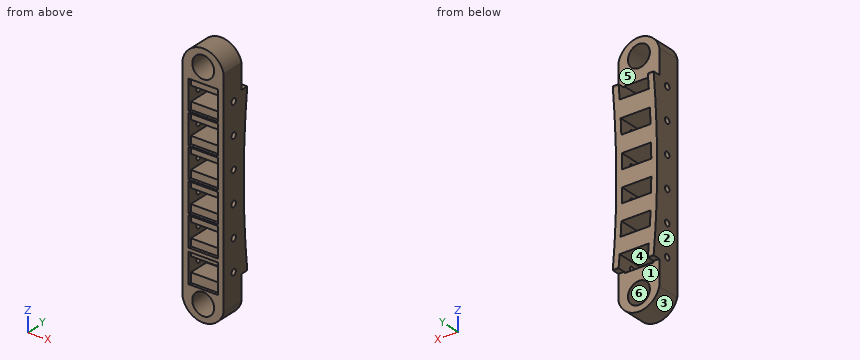
Autodesk Inventor part; units mm, degrees
ref_plane "Work Plane1" through (0, 8.9795, -42.5) normal (0, 1, 0) x (-1, 0, 0)
ref_plane "YZ Plane" through (0, 0, 0) normal (1, 0, 0) x (0, 1, 0)
ref_plane "XY Plane" through (0, 0, 0) normal (0, 0, 1) x (1, 0, 0)
sketch "Sketch1" plane through (0, 0, 0) normal (1, 0, 0) x (0, 1, 0)
  line L0 (0, 0) -> (0, -85)
  line L1 (0, -85) -> (8, -85)
  line L2 (0, 0) -> (8, 0)
  line L3 (8, 0) -> (8, -14)
  line L4 (8, -85) -> (8, -71)
  line L5 (8, -14) -> (9, -14)
  line L6 (8, -71) -> (9, -71)
  arc A0 (10.5, -14.5) -> (10.5, -70.5) centre (267.5593, -42.5) ccw
  line L7 (8, -71) -> (10.555, -71)
  line L8 (8, -14) -> (10.555, -14)
  arc A1 (10.555, -14) -> (10.555, -71) centre (267.5473, -42.5) ccw
extrude "Extrusion1" add sketch "Sketch1" along normal mid plane 14
sketch "Sketch2" plane through (-7, 8, 0) normal (0, 1, 0) x (1, 0, 0)
  line L0 (0, 85) -> (0, 0)
  line L1 (0, 14.0338) -> (0, 5.5338)
  line L2 (14, 0) -> (14, 85)
  line L3 (14, 14.0338) -> (14, 5.5338)
  arc A0 (0, 5.5338) -> (14, 5.5338) centre (7, 7.1942) ccw
  line L4 (0, 5.5338) -> (0, 0)
  line L5 (0, 0) -> (14, 0)
  line L6 (14, 0) -> (14, 5.5338)
  point P0 (7, 0)
  dimension "d13" = 8.5
extrude "Extrusion2" cut sketch "Sketch2" against normal blind 14
sketch "Sketch3" plane through (-7, 8, -71) normal (0, 1, 0) x (1, 0, 0)
  line L0 (0, 0) -> (14, 0)
  line L1 (0, 0) -> (0, 14)
  arc A0 (14, 8.5) -> (0, 8.5) centre (7, 6.7955) ccw
  line L2 (0, 8.5) -> (0, 14)
  line L3 (0, 14) -> (14, 14)
  line L4 (14, 14) -> (14, 8.5)
  line L5 (14, -65.4662) -> (14, 14)
  line L6 (0, 14) -> (0, 8.5)
  line L7 (14, 8.5) -> (14, 14)
  line L8 (14, 14) -> (0, 14)
  line L9 (0, 8.5) -> (0, 14)
  line L10 (0, 14) -> (14, 14)
  line L11 (14, 14) -> (14, 8.5)
  line L12 (14, 14) -> (14, 0)
  arc A1 (14, 8.5) -> (0, 8.5) centre (7, 6.7955) ccw
  point P0 (7, -71)
extrude "Extrusion3" cut sketch "Sketch3" against normal blind 14 contours L1 L3 A0 | A0 L3 L4
sketch "Sketch7" plane through (0, 0, -7.1942) normal (0, -1, 0) x (1, 0, 0)
  circle A0 centre (0, 2.1942) radius 3
  line L0 (0, -0.8058) -> (0, -3.8058)
  circle A1 centre (0, -72.0142) radius 1.5
  line L1 (0, -70.5142) -> (0, -67.5142)
  line L2 (0, -67.5142) -> (-5, -67.5142)
  line L3 (-5, -67.5142) -> (5, -67.5142)
  line L4 (-5, -67.5142) -> (5, -67.5142)
  line L5 (5, -67.5142) -> (5, -57.4342)
  line L6 (5, -57.4342) -> (-5, -57.4342)
  line L7 (-5, -57.4342) -> (-5, -67.5142)
  line L8 (0, -57.4342) -> (0, -56.9342)
  line L9 (-5, -56.2258) -> (5, -56.2258)
  line L10 (5, -56.2258) -> (5, -46.1458)
  line L11 (5, -46.1458) -> (-5, -46.1458)
  line L12 (-5, -46.1458) -> (-5, -56.2258)
  line L13 (0, -46.1458) -> (0, -45.6458)
  line L14 (-5, -45.6458) -> (5, -45.6458)
  line L15 (5, -45.6458) -> (5, -35.5658)
  line L16 (5, -35.5658) -> (-5, -35.5658)
  line L17 (-5, -35.5658) -> (-5, -45.6458)
  line L18 (0, -35.5658) -> (0, -35.0658)
  line L19 (-5, -35.0658) -> (5, -35.0658)
  line L20 (5, -35.0658) -> (5, -24.9858)
  line L21 (5, -24.9858) -> (-5, -24.9858)
  line L22 (-5, -24.9858) -> (-5, -35.0658)
  line L23 (0, -24.9858) -> (0, -24.4858)
  line L24 (-5, -24.4858) -> (5, -24.4858)
  line L25 (5, -24.4858) -> (5, -14.4058)
  line L26 (5, -14.4058) -> (-5, -14.4058)
  line L27 (-5, -14.4058) -> (-5, -24.4858)
  line L28 (0, -14.4058) -> (0, -13.9058)
  line L29 (-5, -13.9058) -> (5, -13.9058)
  line L30 (5, -13.9058) -> (5, -3.8058)
  line L31 (5, -3.8058) -> (-5, -3.8058)
  line L32 (-5, -3.8058) -> (-5, -13.9058)
  point P0 (0, 7.1942)
extrude "Extrusion6" cut sketch "Sketch7" against normal blind 1 contours L31 L30 L29 L32 | L2 L7 L6 L5 L3
sketch "Sketch8" plane through (0, 0, -7.1942) normal (0, -1, 0) x (1, 0, 0)
  line L0 (-5, -57.4342) -> (5, -57.4342)
  line L1 (0, -57.4342) -> (0, -56.9342)
  line L2 (-5, -56.2258) -> (5, -56.2258)
  line L3 (5, -56.2258) -> (5, -46.1458)
  line L4 (5, -46.1458) -> (-5, -46.1458)
  line L5 (-5, -46.1458) -> (-5, -56.2258)
  line L6 (0, -46.1458) -> (0, -45.6458)
  line L7 (-5, -45.6458) -> (5, -45.6458)
  line L8 (5, -45.6458) -> (5, -35.5658)
  line L9 (5, -35.5658) -> (-5, -35.5658)
  line L10 (-5, -35.5658) -> (-5, -45.6458)
  line L11 (0, -35.5658) -> (0, -35.0658)
  line L12 (-5, -35.0658) -> (5, -35.0658)
  line L13 (5, -35.0658) -> (5, -24.9858)
  line L14 (5, -24.9858) -> (-5, -24.9858)
  line L15 (-5, -24.9858) -> (-5, -35.0658)
  line L16 (0, -24.9858) -> (0, -24.4858)
  line L17 (-5, -24.4858) -> (5, -24.4858)
  line L18 (5, -24.4858) -> (5, -14.4058)
  line L19 (5, -14.4058) -> (-5, -14.4058)
  line L20 (-5, -14.4058) -> (-5, -24.4858)
  point P0 (0, 7.1942)
  dimension "d75" = 0.5
  dimension "d76" = 10.08
  dimension "d77" = 0.5
  dimension "d78" = 10.08
  dimension "d79" = 0.5
  dimension "d80" = 10.08
  dimension "d81" = 0.5
  dimension "d82" = 10.08
extrude "Extrusion7" cut sketch "Sketch8" against normal blind 1
sketch "Sketch9" plane through (0, 1, -7.1942) normal (0, -1, 0) x (1, 0, 0)
  line L0 (-5, -67.5142) -> (-5, -57.4342)
  line L1 (5, -57.4342) -> (5, -67.5142)
  line L2 (-5, -59.2658) -> (5, -59.2658)
  line L3 (-5, -64.2658) -> (5, -64.2658)
  line L4 (-5, -64.2658) -> (-5, -59.2658)
  line L5 (5, -64.2658) -> (5, -59.2658)
  line L6 (5, -64.2658) -> (5, -59.2658)
  point P0 (0, 7.1942)
extrude "Extrusion8" cut sketch "Sketch9" against normal blind 20
sketch "Sketch10" plane through (0, 1, -7.1942) normal (0, -1, 0) x (1, 0, 0)
  line L0 (-5, -56.2258) -> (-5, -46.1458)
  line L1 (5, -46.1458) -> (5, -56.2258)
  line L2 (-5, -53.6858) -> (5, -53.6858)
  line L3 (-5, -48.6858) -> (5, -48.6858)
  line L4 (5, -48.6858) -> (5, -53.6858)
  line L5 (-5, -48.6858) -> (-5, -53.6858)
  point P0 (0, 7.1942)
  dimension "d109" = 5
extrude "Extrusion9" cut sketch "Sketch10" against normal blind 20
sketch "Sketch11" plane through (0, 1, -7.1942) normal (0, -1, 0) x (1, 0, 0)
  line L0 (-5, -45.6458) -> (-5, -35.5658)
  line L1 (5, -35.5658) -> (5, -45.6458)
  line L2 (-5, -43.1058) -> (5, -43.1058)
  line L3 (-5, -38.1058) -> (5, -38.1058)
  line L4 (5, -38.1058) -> (5, -43.1058)
  line L5 (-5, -38.1058) -> (-5, -43.1058)
  point P0 (0, 7.1942)
extrude "Extrusion10" cut sketch "Sketch11" against normal blind 20
sketch "Sketch12" plane through (0, 1, -7.1942) normal (0, -1, 0) x (1, 0, 0)
  line L0 (-5, -35.0658) -> (-5, -24.9858)
  line L1 (5, -24.9858) -> (5, -35.0658)
  line L2 (-5, -32.5258) -> (5, -32.5258)
  line L3 (-5, -27.5258) -> (5, -27.5258)
  line L4 (5, -27.5258) -> (5, -32.5258)
  line L5 (-5, -27.5258) -> (-5, -32.5258)
  point P0 (0, 7.1942)
extrude "Extrusion11" cut sketch "Sketch12" against normal blind 20
sketch "Sketch13" plane through (0, 1, -7.1942) normal (0, -1, 0) x (1, 0, 0)
  line L0 (-5, -24.4858) -> (-5, -14.4058)
  line L1 (-5, -21.9458) -> (5, -21.9458)
  line L2 (-5, -16.9458) -> (5, -16.9458)
  line L3 (5, -16.9458) -> (5, -21.9458)
  line L4 (5, -14.4058) -> (5, -24.4858)
  line L5 (-5, -16.9458) -> (-5, -21.9458)
  point P0 (0, 7.1942)
extrude "Extrusion12" cut sketch "Sketch13" against normal blind 20
sketch "Sketch14" plane through (0, 1, -7.1942) normal (0, -1, 0) x (1, 0, 0)
  line L0 (-5, -13.9058) -> (-5, -3.8058)
  line L1 (5, -3.8058) -> (5, -13.9058)
  line L2 (-5, -11.3558) -> (5, -11.3558)
  line L3 (-5, -6.3558) -> (5, -6.3558)
  line L4 (5, -6.3558) -> (5, -11.3558)
  line L5 (-5, -6.772) -> (-5, -11.3558)
  line L6 (-5, -6.3558) -> (-5, -11.3558)
  point P0 (0, 7.1942)
extrude "Extrusion13" cut sketch "Sketch14" against normal blind 20
ref_plane "Work Plane1" through (0, 8.9795, -42.5) normal (0, 1, 0) x (-1, 0, 0)
sketch "Sketch30" plane through (0, 0, -7.1942) normal (0, -1, 0) x (1, 0, 0)
  line L0 (7, 1.6605) -> (7, -72.3058) construction
  line L1 (7, -35.3226) -> (-7, -35.3226) construction
  line L2 (-7, -72.3058) -> (-7, 1.6605) construction
  line L3 (0, -35.3226) -> (0, 1.3774) construction
  line L4 (0, -35.3226) -> (0, -72.0226) construction
  circle A0 centre (0, 1.3774) radius 3.75
  circle A1 centre (0, -72.0226) radius 3.75
  point P0 (0, 7.1942)
  dimension "d140" = 36.7
  dimension "d141" = 36.7
  dimension "d142" = 7.5
  dimension "d143" = 7.5
extrude "Extrusion16" cut sketch "Sketch30" against normal through all
sketch "Sketch31" plane through (7, 0, 0) normal (1, 0, 0) x (0, 0, -1)
  line L0 (13.55, 1) -> (13.55, 8) construction
  line L1 (71.46, 1) -> (71.46, 8) construction
  line L2 (18.55, 1) -> (18.55, 10.0911) construction
  line L3 (24.14, 1) -> (24.14, 9.6322) construction
  line L4 (29.14, 1) -> (29.14, 9.3249) construction
  line L5 (34.72, 1) -> (34.72, 9.0966) construction
  line L6 (39.72, 1) -> (39.72, 8.9945) construction
  line L7 (45.3, 1) -> (45.3, 8.9947) construction
  line L8 (50.3, 1) -> (50.3, 9.0972) construction
  line L9 (55.88, 1) -> (55.88, 9.326) construction
  line L10 (60.88, 1) -> (60.88, 9.6336) construction
  line L11 (66.46, 1) -> (66.46, 10.0921) construction
  line L12 (13.55, 4.5) -> (18.55, 4.5) construction
  line L13 (24.14, 4.5) -> (29.14, 4.5) construction
  line L14 (34.72, 4.5) -> (39.72, 4.5) construction
  line L15 (45.3, 4.5) -> (50.3, 4.5) construction
  line L16 (55.88, 4.5) -> (60.88, 4.5) construction
  line L17 (66.46, 4.5) -> (71.46, 4.5) construction
  circle A0 centre (16.05, 4.5) radius 1
  circle A1 centre (26.64, 4.5) radius 1
  circle A2 centre (37.22, 4.5) radius 1
  circle A3 centre (47.8, 4.5) radius 1
  circle A4 centre (58.38, 4.5) radius 1
  circle A5 centre (68.96, 4.5) radius 1
  point P0 (0, 0)
  dimension "d146" = 2
  dimension "d147" = 2
  dimension "d148" = 2
  dimension "d149" = 2
  dimension "d150" = 2
  dimension "d151" = 2
extrude "Extrusion17" cut sketch "Sketch31" against normal through all
properties part number "Ponte menor" material "Steel"
Check sheet for the modelled part. Datum: model origin and axes. Units: mm. Face numbers are marked on the shaded views. A direction names the side the tool comes from. Round coordinates to 2 decimals unless told otherwise and drop trailing zeros. Order: outer loops, then holes, each group sorted by start corner. A loop starts at its lowest first (then second) coordinate and runs counter-clockwise, first axis right, second up. Notation, with made-up numbers: (-3, 1.5) -> (54, 1.5) arc R12 ccw to (54, 9.5) -> close; hole circle Ø10 at (-35, 44). An arc over 180 degrees is marked (long way). Use CSV: the item, a comma, the result in double quotes.
(1) Material ranges on line 1 along X through (y, z) = (3.75, -18.5); line 2 along Y through (x, z) = (-2.75, -71.5); line 3 along Y through (x, z) = (6.4, -58.38), recorded low to high. Write a range as from..to.
Worked out:
line 1,"-7..-5, 5..7"
line 2,"1..8"
line 3,"0..3.5, 5.5..9.47"
(2) Depth check by flat-ended pin: pin 1 (2.5 mm diameter, centred on x = 1.5, y = 7, fed in from -Z); pin 2 (0.8 mm diameter, centred on x = -1.5, y = 0.5, fed in from +Z); pin 3 (2.5 mm diameter, centred on y = 4.5, z = -16.05, fed in from -X); pin 4 (2 mm diameter, centred on x = -3.5, y = 5.5, fed in from +Z). Enter the tip coordinate at first touch or a pass-through.
Worked out:
pin 1,"z = -85"
pin 2,"z = -0.08"
pin 3,"x = -7"
pin 4,"z = -0.45"
(3) Cross-section at C-C (z = -16.05). Record the boundary of the cut face in (x, y), and give its area (3 significant figures).
Worked out:
outline,"(-7, 0) -> (-5, 0) -> (-5, 3.5) -> (-7, 3.5) -> close; (-7, 5.5) -> (-5, 5.5) -> (-5, 10.34) -> (-7, 10.34) -> close; (5, 0) -> (7, 0) -> (7, 3.5) -> (5, 3.5) -> close; (5, 5.5) -> (7, 5.5) -> (7, 10.34) -> (5, 10.34) -> close"
area,"33.3 mm²"
(4) Draft check along X on the marked faces 1, 2, 3 and 4. Enter one of: pulls with the +X half, pulls with the -X half, needs draft (parallel to the pull), parting line crosses it, or undercut.
Worked out:
face 1,"needs draft"
face 2,"pulls with the -X half"
face 3,"parting line crosses it"
face 4,"undercut"
(5) Cross-section at B-B (x = 0). Count the separate pieces of the cut face and the enclosed holes in it, and give its area (3 significant figures).
Worked out:
separate pieces,"9"
enclosed holes,"0"
area,"329 mm²"
(6) Tool access check on the marked faces 5 and 6. Record the directions out of +Z, -Z, +X, -X, +Y, -Y that give a thin tool (end or side, any length) a straight path to the whole face; none if there is none.
Worked out:
face 5,"+Z, +X, -X, +Y"
face 6,"+Y, -Y"
(7) Cross-section at A-A (z = -37.22). Record the boundary of the cut face in (x, y).
Worked out:
outline,"(-7, 0) -> (-5, 0) -> (-5, 3.5) -> (-7, 3.5) -> close; (-7, 5.5) -> (-5, 5.5) -> (-5, 9.03) -> (-7, 9.03) -> close; (5, 0) -> (7, 0) -> (7, 3.5) -> (5, 3.5) -> close; (5, 5.5) -> (7, 5.5) -> (7, 9.03) -> (5, 9.03) -> close"
